```python
from build123d import *

# Parameters (mm, degrees)
CIRCLE_R         = 3.75
EXTRUDE001_DEPTH = 1.5
CIRCLE001_R      = 3
EXTRUDE_DEPTH    = 10
BOX_W            = 7.5
BOX_H            = 7.5
BOX_DEPTH        = 1


with BuildPart() as extrude001:
    # Circle → Extrude001 (new body)
    with BuildSketch(Plane(origin=(3.75, 3.75, 1), x_dir=(-1, 0, 0), z_dir=(0, 0, 1))):
        Circle(CIRCLE_R)
    extrude(amount=EXTRUDE001_DEPTH)


with BuildPart() as extrude001_1:
    # Extrude001 placement: moved
    add(extrude001.part.moved(Location((0, 0, -1.5))))


with BuildPart() as fusion:
    # Circle001 → Extrude (new body)
    with BuildSketch(Plane(origin=(3.75, 3.75, 1), x_dir=(-1, 0, 0), z_dir=(0, 0, 1))):
        Circle(CIRCLE001_R)
    extrude(amount=EXTRUDE_DEPTH)


with BuildPart() as fusion_1:
    # Extrude placement: moved
    add(fusion.part.moved(Location((0, 0, -10))))

    # Fusion: union Extrude001
    add(extrude001_1.part)


with BuildPart() as obj1:
    # Box → Box (new body)
    with BuildSketch(Plane.XY):
        with Locations((3.75, 3.75)):
            Rectangle(BOX_W, BOX_H)
    extrude(amount=BOX_DEPTH)

    # Fusion001: union Fusion
    add(fusion_1.part)


solid = obj1.part
```
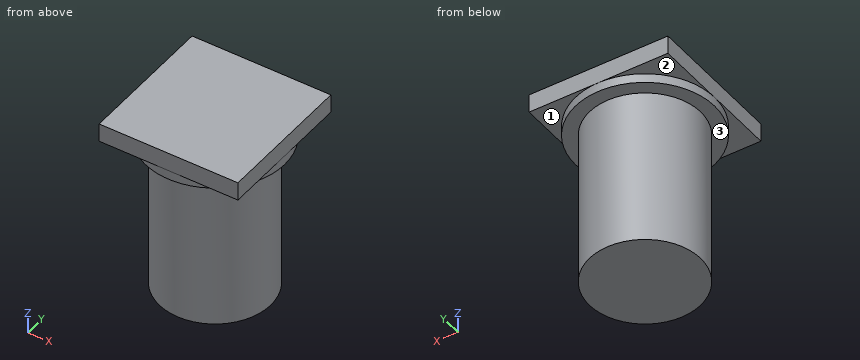
Work out the finished part from the listing and answer in its coordinate system (mm). Face numbers are marked on the shaded views. A direction names the side the tool comes from. Give positions to 0.01 mm unless a question says otherwise; leave off trailing zeros. Loops run counter-clockwise (first coordinate to the right, second up) from the corner with the lowest first, then second, coordinate; pieces in that order, holes last. Notation, with made-up numbers: (55, -30.75) -> (63, -30.75) arc R30 cw to (63, 2.25) -> close; hole circle Ø10 at (12, 42.25). An arc over 180 degrees is marked (long way). Use CSV: the item, a comma, the result in double quotes.
1. The part is cut by section B-B (z = -4). Write down the section's boundary in (x, y), then the cut area to 3 significant figures.
Found:
outline,"circle Ø6 at (3.75, 3.75)"
area,"28.3 mm^2"
2. The part is cut by section C-C (y = 5.5). Write down the section's boundary in (x, z).
Found:
outline,"(0, 0) -> (0.43, 0) -> (0.43, -0.5) -> (1.31, -0.5) -> (1.31, -9) -> (6.19, -9) -> (6.19, -0.5) -> (7.07, -0.5) -> (7.07, 0) -> (7.5, 0) -> (7.5, 1) -> (0, 1) -> close"
3. Straight lines are drawn through the part: line 1 (X direction, y = 3.75, z = -1); line 2 (Z direction, x = 6.75, y = 1.75). For each, find the intervals that lie inside material, in ascending order.
Found:
line 1,"0.75 to 6.75"
line 2,"-0.5 to 1"
4. A tool of negligible diameter and unlimited length cuts with its end or side. For the marked faces 1, 2 and 3, from which of +Z, -Z, +X, -X, +Y, -Y can it reach the whole face along a straight path? Write none if from no direction.
Found:
face 1,"-Z, +X, +Y"
face 2,"-Z, -X, +Y"
face 3,"-Z"
5. The part is cut by section A-A (x = 5). Write down the section's boundary in (y, z), then the cut area to 3 significant figures.
Found:
outline,"(0, 0) -> (0.21, 0) -> (0.21, -0.5) -> (1.02, -0.5) -> (1.02, -9) -> (6.48, -9) -> (6.48, -0.5) -> (7.29, -0.5) -> (7.29, 0) -> (7.5, 0) -> (7.5, 1) -> (0, 1) -> close"
area,"57.4 mm^2"
6. A flat-ended cylindrical pin translates along its axis: pin 1 Ø1.5 at (x, z) = (5.5, -6.5) entering from +Y. Find the tip coordinate at first contact, or state that the pin passes through.
Found:
pin 1,"y = 6.58"
